For this review, take the finished solid that the model builds, in its own axes (mm). A direction names the side the tool comes from. Coordinates: 2 decimals unless noted, no trailing zeros. Loops run counter-clockwise (first coordinate to the right, second up) from the corner with the lowest first, then second, coordinate; pieces in that order, holes last. Notation, with made-up numbers: M 41,25 L 74,25 A12 cw 74,42 Z; hole C 80,14.5 d1. An arc over 180 degrees is marked long. Write item = value, one per line.
from build123d import *

# Parameters (mm, degrees)
F3_R      = 12.7
F4_DEPTH  = 64.501
F5_DEPTH  = 73
F6_R      = 7.62
F7_DEPTH  = 73.001
F8_W      = 30
F8_H      = 4.40173278
F9_DEPTH  = 8.5
F12_D     = 3.3
F12_DEPTH = 30
F12_TIP   = 0.9914200214


with BuildPart() as f1:
    # F0 (on Front) → F1 (revolve)
    with BuildSketch(Plane.XZ):
        with BuildLine():
            Line((0, -28.1334591306), (0, 27.8665408694))
            Line((0, 27.8665408694), (-35, 27.8665408694))
            Line((-35, 27.8665408694), (-35, 21.8665408694))
            ThreePointArc((-35, 21.8665408694), (-23, -0.1334591306), (-35, -22.1334591306))
            Line((-35, -22.1334591306), (-35, -28.1334591306))
            Line((-35, -28.1334591306), (0, -28.1334591306))
        make_face()
    revolve(axis=Axis((0, 0, -0.1334591306), (0, 0, -1)))

    # F3 (on offset) → F4 (cut, through all)
    with BuildSketch(Plane.XY.offset(36.3665408694)):
        Circle(F3_R)
    extrude(amount=-F4_DEPTH, mode=Mode.SUBTRACT)

    # F3 (on offset) → F5 (join)
    with BuildSketch(Plane.XY.offset(36.3665408694)):
        Circle(F3_R)
    extrude(amount=-F5_DEPTH)

    # F6 (on face) → F7 (cut, through all)
    with BuildSketch(Plane.XY.offset(36.3665408694)):
        Circle(F6_R)
    extrude(amount=-F7_DEPTH, mode=Mode.SUBTRACT)

    # F8 (on face) → F9 (cut)
    with BuildSketch(Plane.XY.offset(36.3665408694)):
        with Locations((0, -11.20086639)):
            Rectangle(F8_W, F8_H)
        Polygon((-15, 9), (15, 9), (15.7737210393, 16.7225152254), (-15, 16.7225152254), align=None)
    extrude(amount=-F9_DEPTH, mode=Mode.SUBTRACT)

    # F12
    with Locations(Plane.YZ.offset(12.7)):
        with Locations((0, 32.1165408694)):
            Hole(F12_D / 2, depth=F12_DEPTH)
            with Locations((0, 0, -(F12_DEPTH + F12_TIP / 2))):  # 118° drill point
                Cone(0, F12_D / 2, F12_TIP, mode=Mode.SUBTRACT)


solid = f1.part
Q1. For pin 1 Ø4 at (x, y) = (-24, -20) entering from -Z; pin 2 Ø2 at (y, z) = (20, 7) entering from -X; pin 3 Ø5.5 at (y, z) = (0, 32.12) entering from -X; pin 4 Ø9 at (x, y) = (0, 0) entering from +Z, all flat-tipped, find the tip position at first contact; note any pin that passes through.
Solved:
pin_1 = -28.13
pin_2 = -14.73
pin_3 = -12.7
pin_4 = through
Q2. Draft analysis for pull direction Y (two halves, no side actions). For faces 1 (the face through (28, -21, 25)), 2 (the face through (-10.1, -0.9, 33.5)), 3 (the face through (0, -15, 27.867)), state which applies: +Y half, -Y half, draft (parallel to the pull), parting line (faces both ways), or undercut.
Solved:
face_1 = parting line
face_2 = undercut
face_3 = draft
Q3. Add section B-B (x = 0). Write out the cut boundary in (y, z).
Solved:
outline = M -35,-28.13 L -12.7,-28.13 L -12.7,-36.63 L -7.62,-36.63 L -7.62,36.37 L -9,36.37 L -9,27.87 L -35,27.87 L -35,21.87 A26.17 cw -35,-22.13 Z; M 7.62,-36.63 L 12.7,-36.63 L 12.7,-28.13 L 35,-28.13 L 35,-22.13 A26.17 cw 35,21.87 L 35,27.87 L 9,27.87 L 9,36.37 L 7.62,36.37 Z
Q4. Machinability: for faces 4 (the face through (-12.7, 0.1, 30.3)), 5 (the face through (0, -15, -28.133)), 6 (the face through (0, 9, 32)), 7 (the face through (12.7, -0.1, 30.3)), 8 (the face through (0, -9, 32)), which of the approach directions +Z, -Z, +X, -X, +Y, -Y give a long, thin tool a straight path to every point of the face, cutting with its end or side? Answer none if there is none.
Solved:
face_4 = +Z, -X
face_5 = -Z
face_6 = +Z, +X, -X, +Y
face_7 = +Z, +X
face_8 = +Z, +X, -X, -Y
Q5. For line 1 along Z through (x, y) = (15.5, -7); line 2 along Z through (x, y) = (6.5, 26); line 3 along Z through (x, y) = (8.9, 0), list the stretches that pass through material, from the lowest coordinate up.
Solved:
line_1 = -28.13 to 27.87
line_2 = -28.13 to -13.71, 13.45 to 27.87
line_3 = -36.63 to 30.47, 33.77 to 36.37
Q6. Add section C-C (z = 23). Write out the cut boundary in (x, y).
Solved:
outline = C 0,0 d70; hole C 0,0 d15.24
Q7. Add section A-A (y = 0). Write out the cut boundary in (x, z), and give its area (3 significant figures).
Solved:
outline = M -35,-28.13 L -12.7,-28.13 L -12.7,-36.63 L -7.62,-36.63 L -7.62,30.47 L -12.7,30.47 L -12.7,27.87 L -35,27.87 L -35,21.87 A26.17 cw -35,-22.13 Z; M -12.7,33.77 L -7.62,33.77 L -7.62,36.37 L -12.7,36.37 Z; M 7.62,-36.63 L 12.7,-36.63 L 12.7,-28.13 L 35,-28.13 L 35,-22.13 A26.17 cw 35,21.87 L 35,27.87 L 12.7,27.87 L 12.7,30.47 L 7.62,30.47 Z; M 7.62,33.77 L 12.7,33.77 L 12.7,36.37 L 7.62,36.37 Z
area = 2,460 mm²
Q8. Add section D-D (z = 8). Write out the cut boundary in (x, y).
Solved:
outline = C 0,0 d48.59; hole C 0,0 d15.24
